from build123d import *

# Parameters (mm, degrees)
SKETCH_1_R      = 2
EXTRUDE_1_DEPTH = 1
SKETCH_1_3_R    = 12
SKETCH_1_3_R_2  = 10.130489444
SKETCH_1_3_R_3  = 6
EXTRUDE_2_DEPTH = 12


with BuildPart() as part:
    # Sketch 1 → Extrude 1 (new body)
    with BuildSketch(Plane(origin=(0, 0, 0), x_dir=(1, 0, 0), z_dir=(0, 1, 0))):
        with BuildLine():
            ThreePointArc((-20.357142857, 4.103259033), (-22.5, 0), (-20.357142857, -4.103259033))
            Line((-20.357142857, -4.103259033), (-8.571428571, -12.3097771))
            ThreePointArc((-8.571428571, -12.3097771), (0, -15), (8.571428571, -12.3097771))
            Line((8.571428571, -12.3097771), (20.357142857, -4.103259033))
            ThreePointArc((20.357142857, -4.103259033), (22.5, 0), (20.357142857, 4.103259033))
            Line((20.357142857, 4.103259033), (8.571428571, 12.3097771))
            ThreePointArc((8.571428571, 12.3097771), (0, 15), (-8.571428571, 12.3097771))
            Line((-8.571428571, 12.3097771), (-20.357142857, 4.103259033))
        make_face()
        with Locations(Location((-17.5, 0, 0), (0, 0, 270))):
            Circle(SKETCH_1_R, mode=Mode.SUBTRACT)
        with Locations(Location((17.5, 0, 0), (0, 0, 270))):
            Circle(SKETCH_1_R, mode=Mode.SUBTRACT)
    extrude(amount=EXTRUDE_1_DEPTH)

    # Sketch 1_3 → Extrude 2 (add)
    # profile 1 of 2: a face of its own
    with BuildSketch(Plane(origin=(0, 0, 0), x_dir=(1, 0, 0), z_dir=(0, 1, 0))):
        with Locations(Location((0, 0, 0), (0, 0, 270))):
            Circle(SKETCH_1_3_R)
        Circle(SKETCH_1_3_R_2, mode=Mode.SUBTRACT)
    # profile 2 of 2: a face of its own
    with BuildSketch(Plane(origin=(0, 0, 0), x_dir=(1, 0, 0), z_dir=(0, 1, 0))):
        Circle(SKETCH_1_3_R_2)
        with Locations(Location((0, 0, 0), (0, 0, 270))):
            Circle(SKETCH_1_3_R_3, mode=Mode.SUBTRACT)
    extrude(amount=EXTRUDE_2_DEPTH)


solid = part.part
Verification items for the finished model (mm, model axes). A direction names the side the tool comes from. Give positions to 0.01 mm unless a question says otherwise; leave off trailing zeros. Order: outer loops, then holes, each group sorted by start corner. A loop starts at its lowest first (then second) coordinate and runs counter-clockwise, first axis right, second up. Notation, with made-up numbers: M 1.25,58 L 52.25,58 A6 ccw 52.25,62 Z; hole C 79,88.5 d9. An arc over 180 degrees is marked long. Answer as a JSON object with one key per item and string values. Group by question number.
1) Cross-section at D-D (y = 8.25). Enter the section's corners in (x, z), then the cut area to 3 significant figures.
2) Cross-section at A-A (z = 0). Enter the section's corners in (x, y).
3) Depth check by flat-ended pin: pin 1 Ø4 at (x, y) = (-6, 5) entering from -Z; pin 2 Ø9.5 at (x, z) = (0.5, 1) entering from +Y. Enter the tip coordinate at first touch or a pass-through.
4) Access from +Z, -Z, +X, -X, +Y, -Y to the whole of each face (thin tool, end or side, straight path). Record for faces 4 (the face through (0, 0, 0)), 5 (the face through (3.604, 6.423, 11.446)).
5) Cross-section at C-C (x = 0). Enter the section's corners in (y, z), then the cut area to 3 significant figures.
6) Mould release check, pull along Z, two halves, no side actions. Record for faces 1 (the face through (22.5, 0.5, 0.1)), 2 (the face through (-14.382, 0.493, -8.264)), 3 (the face through (0, 1, 0)): released by +Z, released by -Z, zero draft, split by the parting line, or undercut.
7) Scan lines: line 1 along X through (y, z) = (0.5, 0); line 2 along X through (y, z) = (4, 0). Record each from-to range of solid material in increasing order. Write a range as [from, to].
8) Cross-section at B-B (x = -18). Enter the section's corners in (y, z), then the cut area to 3 significant figures.
Result sheet:
{
 "1": {"outline": "C 0,0 d24; hole C 0,0 d12", "area": "339 mm2"},
 "2": {"outline": "M -22.5,0 L -19.5,0 L -19.5,1 L -22.5,1 Z; M -15.5,0 L 15.5,0 L 15.5,1 L 12,1 L 12,12 L 6,12 L 6,1 L -6,1 L -6,12 L -12,12 L -12,1 L -15.5,1 Z; M 19.5,0 L 22.5,0 L 22.5,1 L 19.5,1 Z"},
 "3": {"pin 1": "stops at z = -11.31", "pin 2": "stops at y = 1"},
 "4": {"face 4": "+Z, -Z, +X, -X, -Y", "face 5": "+Y"},
 "5": {"outline": "M 0,-15 L 1,-15 L 1,-12 L 12,-12 L 12,-6 L 1,-6 L 1,6 L 12,6 L 12,12 L 1,12 L 1,15 L 0,15 Z", "area": "162 mm2"},
 "6": {"face 1": "split by the parting line", "face 2": "released by -Z", "face 3": "undercut"},
 "7": {"line 1": "x = [-22.5, -19.5], [-15.5, 15.5], [19.5, 22.5]", "line 2": "x = [-12, -6], [6, 12]"},
 "8": {"outline": "M 0,-5.74 L 1,-5.74 L 1,-1.94 L 0,-1.94 Z; M 0,1.94 L 1,1.94 L 1,5.74 L 0,5.74 Z", "area": "7.62 mm2"}
}
